Input: part model. Units: mm. Frame: model coordinates. Face numbers are marked on the shaded views. A direction names the side the tool comes from. Round coordinates to 2 decimals unless told otherwise and drop trailing zeros. Order: outer loops, then holes, each group sorted by start corner. A loop starts at its lowest first (then second) coordinate and runs counter-clockwise, first axis right, second up. Notation, with made-up numbers: (-12, -8) -> (0, -8) arc R7 ccw to (0, 4) -> close; hole circle Ø10 at (30, -10.5). An arc over 180 degrees is marked (long way). Use a Markdown table: item, result.
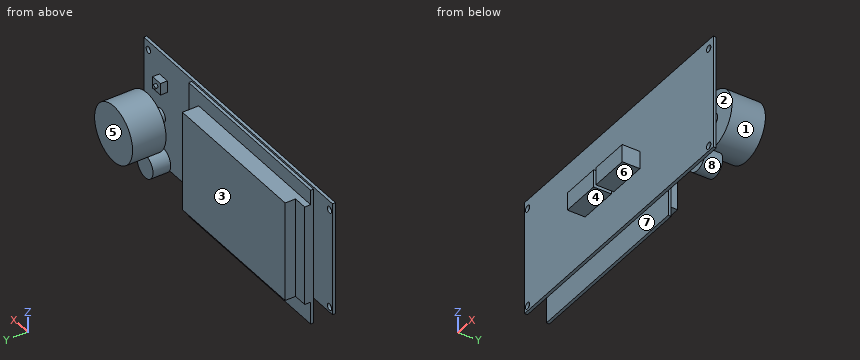
from build123d import *

# Parameters (mm, degrees)
SKETCH1_W            = 144
SKETCH1_H            = 58
BOSS_EXTRUDE2_DEPTH  = 1.5
SKETCH2_W            = 93
SKETCH2_H            = 70
BOSS_EXTRUDE3_DEPTH  = 1.5
SKETCH3_W            = 78.4
SKETCH3_H            = 51
BOSS_EXTRUDE4_DEPTH  = 8.3
SKETCH4_W            = 7
SKETCH4_H            = 51
BOSS_EXTRUDE5_DEPTH  = 3
SKETCH5_R            = 3.5
BOSS_EXTRUDE6_DEPTH  = 7
SKETCH6_R            = 14.5
BOSS_EXTRUDE7_DEPTH  = 17
SKETCH8_R            = 6
BOSS_EXTRUDE8_DEPTH  = 9
SKETCH9_W            = 6
SKETCH9_H            = 6
BOSS_EXTRUDE9_DEPTH  = 3.5
SKETCH10_R           = 1.016941324
BOSS_EXTRUDE10_DEPTH = 1.5
SKETCH11_W           = 20
SKETCH11_H           = 9
BOSS_EXTRUDE11_DEPTH = 9
SKETCH12_R           = 1.65
CUT_EXTRUDE2_DEPTH   = 10


with BuildPart() as part:
    # Sketch1 → Boss-Extrude2 (new body)
    with BuildSketch(Plane(origin=(0, 0, 0), x_dir=(1, 0, 0), z_dir=(0, 1, 0))):
        Rectangle(SKETCH1_W, SKETCH1_H)
    extrude(amount=BOSS_EXTRUDE2_DEPTH)

    # Sketch2 → Boss-Extrude3 (add)
    with BuildSketch(Plane(origin=(0, 1.5, 0), x_dir=(1, 0, 0), z_dir=(0, 1, 0))):
        with Locations((-11.1, 7)):
            Rectangle(SKETCH2_W, SKETCH2_H)
    extrude(amount=BOSS_EXTRUDE3_DEPTH)

    # Sketch3 → Boss-Extrude4 (add)
    with BuildSketch(Plane(origin=(0, 3, 0), x_dir=(1, 0, 0), z_dir=(0, 1, 0))):
        with Locations((-11.4, 5.076084889)):
            Rectangle(SKETCH3_W, SKETCH3_H)
    extrude(amount=BOSS_EXTRUDE4_DEPTH)

    # Sketch4 → Boss-Extrude5 (add)
    with BuildSketch(Plane(origin=(0, 3, 0), x_dir=(1, 0, 0), z_dir=(0, 1, 0))):
        with Locations((-54.1, 5.076084889)):
            Rectangle(SKETCH4_W, SKETCH4_H)
    extrude(amount=BOSS_EXTRUDE5_DEPTH)

    # Sketch5 → Boss-Extrude6 (add)
    with BuildSketch(Plane(origin=(0, 1.5, 0), x_dir=(1, 0, 0), z_dir=(0, 1, 0))):
        with Locations(Location((59, 4, 0), (0, 0, 90))):
            Circle(SKETCH5_R)
    extrude(amount=BOSS_EXTRUDE6_DEPTH)

    # Sketch6 → Boss-Extrude7 (add)
    with BuildSketch(Plane(origin=(0, 8.5, 0), x_dir=(1, 0, 0), z_dir=(0, 1, 0))):
        with Locations(Location((59, 4, 0), (0, 0, 270))):
            Circle(SKETCH6_R)
    extrude(amount=BOSS_EXTRUDE7_DEPTH)

    # Sketch8 → Boss-Extrude8 (add)
    with BuildSketch(Plane(origin=(0, 1.5, 0), x_dir=(1, 0, 0), z_dir=(0, 1, 0))):
        with Locations(Location((57.45, 26, 0), (0, 0, 150))):
            Circle(SKETCH8_R)
    extrude(amount=BOSS_EXTRUDE8_DEPTH)

    # Sketch9 → Boss-Extrude9 (add)
    with BuildSketch(Plane(origin=(0, 1.5, 0), x_dir=(1, 0, 0), z_dir=(0, 1, 0))):
        with Locations((57, -14)):
            Rectangle(SKETCH9_W, SKETCH9_H)
    extrude(amount=BOSS_EXTRUDE9_DEPTH)

    # Sketch10 → Boss-Extrude10 (add)
    with BuildSketch(Plane(origin=(0, 5, 0), x_dir=(1, 0, 0), z_dir=(0, 1, 0))):
        with Locations(Location((57, -14, 0), (0, 0, 270))):
            Circle(SKETCH10_R)
    extrude(amount=BOSS_EXTRUDE10_DEPTH)

    # Sketch11 → Boss-Extrude11 (add)
    with BuildSketch(Plane.XZ):
        with Locations((6, -2)):
            Rectangle(SKETCH11_W, SKETCH11_H)
        with Locations((-15.8, -2)):
            Rectangle(SKETCH11_W, SKETCH11_H)
    extrude(amount=BOSS_EXTRUDE11_DEPTH)

    # Sketch12 → Cut-Extrude2 (cut)
    with BuildSketch(Plane(origin=(0, 0, 0), x_dir=(1, 0, 0), z_dir=(0, 1, 0))):
        with Locations(Location((68.5, 26.3, 0), (0, 0, 90))):
            Circle(SKETCH12_R)
        with Locations(Location((68.5, -24.5, 0), (0, 0, 90))):
            Circle(SKETCH12_R)
        with Locations(Location((-69.75, 26.3, 0), (0, 0, 90))):
            Circle(SKETCH12_R)
        with Locations(Location((-69.75, -24.5, 0), (0, 0, 90))):
            Circle(SKETCH12_R)
    extrude(amount=CUT_EXTRUDE2_DEPTH, mode=Mode.SUBTRACT)


solid = part.part
1) Cut plane B-B on z = -11. Return loops of the section in (x, y), and give its area (3 significant figures).
Results found:
| item | result |
|---|---|
| outline | (-72, 0) -> (72, 0) -> (72, 1.5) -> (35.4, 1.5) -> (35.4, 3) -> (27.8, 3) -> (27.8, 11.3) -> (-50.6, 11.3) -> (-50.6, 6) -> (-57.6, 6) -> (-57.6, 1.5) -> (-72, 1.5) -> close; (46.3, 8.5) -> (71.7, 8.5) -> (71.7, 25.5) -> (46.3, 25.5) -> close |
| area | 1,460 mm² |
2) Cut plane A-A on x = -69.75. Return loops of the section in (y, z).
Results found:
| item | result |
|---|---|
| outline | (0, -29) -> (1.5, -29) -> (1.5, -27.95) -> (0, -27.95) -> close; (0, -24.65) -> (1.5, -24.65) -> (1.5, 22.85) -> (0, 22.85) -> close; (0, 26.15) -> (1.5, 26.15) -> (1.5, 29) -> (0, 29) -> close |
3) Cut plane D-D on x = -30. Return loops of the section in (y, z), and give its area (3 significant figures).
Results found:
| item | result |
|---|---|
| outline | (0, -29) -> (1.5, -29) -> (1.5, -42) -> (3, -42) -> (3, -30.58) -> (11.3, -30.58) -> (11.3, 20.42) -> (3, 20.42) -> (3, 28) -> (1.5, 28) -> (1.5, 29) -> (0, 29) -> close |
| area | 615 mm² |
4) Pull-direction query (Z, two-part tool) for the marked faces 6, 7 and 8; classes: +Z half, -Z half, draft (parallel to the pull), parting line (faces both ways), or undercut.
Results found:
| item | result |
|---|---|
| face 6 | -Z half |
| face 7 | draft |
| face 8 | undercut |
5) Pin query (flat end, axial travel): pin 1 Ø3.5 at (y, z) = (5, -12) entering from -X; pin 2 Ø4 at (y, z) = (10, -7.5) entering from -X; pin 3 Ø1.5 at (x, y) = (-19.5, 5.5) entering from +Z; pin 4 Ø6.5 at (x, z) = (58.5, 13) entering from +Y. Return the tip coordinate at first contact, or that it passes through.
Results found:
| item | result |
|---|---|
| pin 1 | stops at x = -57.6 |
| pin 2 | stops at x = -50.6 |
| pin 3 | stops at z = 20.42 |
| pin 4 | stops at y = 25.5 |
6) Set-up query: the marked faces 1, 2, 3, 4 and 5. Return all of +Z, -Z, +X, -X, +Y, -Y with unobstructed straight access to the full face (end or side cutting, diameter ignored); none if empty.
Results found:
| item | result |
|---|---|
| face 1 | +Y |
| face 2 | none |
| face 3 | +Z, -Z, -X, +Y |
| face 4 | -Z, +X, -X, -Y |
| face 5 | +Z, -Z, +X, -X, +Y |
7) Line query: L1, parallel to Z at x = -69.75, y = 1; L2, parallel to X at y = 0.3, z = -26.3; L3, parallel to Z at x = 4, y = -2. Output: solid intervals per line, ascending. Write a range as [from, to].
Results found:
| item | result |
|---|---|
| L1 | z = [-29, -27.95], [-24.65, 22.85], [26.15, 29] |
| L2 | x = [-72, -71.4], [-68.1, 66.85], [70.15, 72] |
| L3 | z = [-6.5, 2.5] |
8) Cut plane C-C on y = -2. Return loops of the section in (x, z).
Results found:
| item | result |
|---|---|
| outline | (-25.8, -6.5) -> (-5.8, -6.5) -> (-5.8, 2.5) -> (-25.8, 2.5) -> close; (-4, -6.5) -> (16, -6.5) -> (16, 2.5) -> (-4, 2.5) -> close |
